Part model, mm, in its own coordinate system. Face numbers are marked on the shaded views. A direction names the side the tool comes from. Round coordinates to 2 decimals unless told otherwise and drop trailing zeros. Write each loop counter-clockwise with the first axis right and the second up, starting at its lowest first coordinate (ties: lowest second). Pieces come first, ordered by that corner, then holes.
1) Flat gauge pins, fed straight in: pin 1 (3 mm diameter, centred on x = 26.5, y = 5.5, fed in from +Z); pin 2 (2.5 mm diameter, centred on y = 7.5, z = 14.5, fed in from -X); pin 3 (2 mm diameter, centred on x = 33, y = 6, fed in from +Z). Where does each tip first touch, or does it go through?
2) Pull direction X, two halves, no side cores. Call the marked faces 1, 2 and 3: +X half, -X half, draft (parallel to the pull), parting line (faces both ways), or undercut.
3) Saw through at A-A on y = 6. Write the cut outline in (x, z), and give its area (3 significant figures).
4) Drill centre lines: L1, parallel to X at y = 6, z = 2.6; L2, parallel to X at y = 3.5, z = 14; L3, parallel to Y at x = 5, z = 3.2. Where is each one in solid material? Low to high.
5) Saw through at B-B on x = 31. Write the cut outline in (y, z).
6) Which spindle directions (+Z, -Z, +X, -X, +Y, -Y) get a long thin tool onto all of the face, cutting with end or side? Do the marked faces 4 and 5. Say none if no direction does.
7) Saw through at D-D on z = 2.75. Write the cut outline in (x, y).
8) Saw through at C-C on z = 14. Write the cut outline in (x, y).
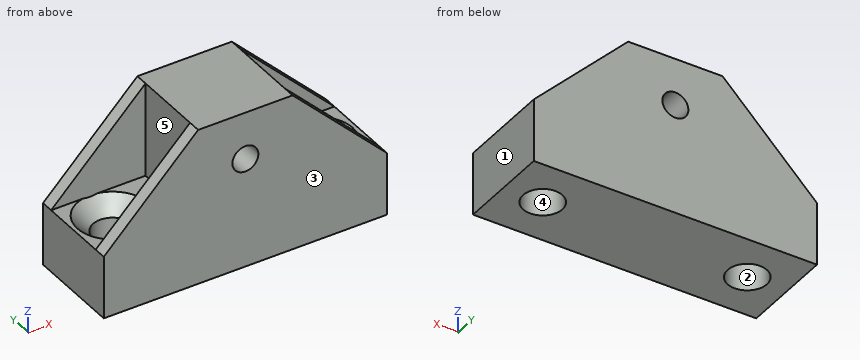
```python
from build123d import *

# Parameters (mm, degrees)
ESQUISSE1_W                  = 36
ESQUISSE1_H                  = 12
BOSS_EXTRU_1_DEPTH           = 8
ENL_V_MAT_EXTRU_1_DEPTH      = 39.781438859
ENL_V_MAT_EXTRU_1_DEPTH_BACK = 39.781438859
ESQUISSE2_R                  = 2.5
ESQUISSE3_W                  = 12
ESQUISSE3_H                  = 12
BOSS_EXTRU_2_DEPTH           = 12
ENL_V_MAT_EXTRU_2_DEPTH      = 43.895221179
ENL_V_MAT_EXTRU_2_DEPTH_BACK = 43.895221179
ESQUISSE4_R                  = 1.65
BOSS_EXTRU_3_DEPTH           = 1.6
BOSS_EXTRU_4_START           = -12
BOSS_EXTRU_4_DEPTH           = 1.6
CHANFREIN1_SIZE              = 2


with BuildPart() as part:
    # Esquisse1 → Boss.-Extru.1 (new body)
    with BuildSketch(Plane.XY):
        with Locations((18, 6)):
            Rectangle(ESQUISSE1_W, ESQUISSE1_H)
    extrude(amount=BOSS_EXTRU_1_DEPTH)

    # Esquisse2 → Enlèv. mat.-Extru.1 (cut, two sides: drawn at the far end of the back side and taken through both)
    with BuildSketch(Plane.XY.offset(8).offset(-ENL_V_MAT_EXTRU_1_DEPTH_BACK)):
        with Locations((5, 6)):
            Circle(ESQUISSE2_R)
        with Locations(Location((31, 6, 0), (0, 0, 180))):
            Circle(ESQUISSE2_R)
    extrude(amount=ENL_V_MAT_EXTRU_1_DEPTH + ENL_V_MAT_EXTRU_1_DEPTH_BACK, mode=Mode.SUBTRACT)

    # Esquisse3 → Boss.-Extru.2 (add)
    with BuildSketch(Plane(origin=(0, 12, 0), x_dir=(1, 0, 0), z_dir=(0, 1, 0))):
        with Locations((18, -14)):
            Rectangle(ESQUISSE3_W, ESQUISSE3_H)
    extrude(amount=-BOSS_EXTRU_2_DEPTH)

    # Esquisse4 → Enlèv. mat.-Extru.2 (cut, two sides: drawn at the far end of the back side and taken through both)
    with BuildSketch(Plane(origin=(0, 12, 0), x_dir=(1, 0, 0), z_dir=(0, 1, 0)).offset(-ENL_V_MAT_EXTRU_2_DEPTH_BACK)):
        with Locations(Location((18, -14, 0), (0, 0, 270))):
            Circle(ESQUISSE4_R)
    extrude(amount=ENL_V_MAT_EXTRU_2_DEPTH + ENL_V_MAT_EXTRU_2_DEPTH_BACK, mode=Mode.SUBTRACT)

    # Esquisse5 → Boss.-Extru.3 (add)
    with BuildSketch(Plane.XZ):
        Polygon((12, 8), (0, 8), (12, 20), align=None)
        Polygon((24, 20), (24, 8), (36, 8), align=None)
    extrude(amount=-BOSS_EXTRU_3_DEPTH)

    # Esquisse5<2> → Boss.-Extru.4 (add)
    with BuildSketch(Plane.XZ.offset(BOSS_EXTRU_4_START)):
        Polygon((12, 8), (0, 8), (12, 20), align=None)
        Polygon((24, 20), (24, 8), (36, 8), align=None)
    extrude(amount=BOSS_EXTRU_4_DEPTH)

    # Chanfrein1
    # the kernel refuses this chamfer: 2 mm, written as the material it takes off along each edge
    with BuildSketch(Plane(origin=(5, 6, 8), x_dir=(1, 0, 0), z_dir=(0, -1, 0))) as chanfrein1_piece_1_section:
        Polygon((2.5 + CHANFREIN1_SIZE, 0), (2.5, -CHANFREIN1_SIZE), (2.5, 0), align=None)
    chanfrein1_piece_1 = revolve(axis=Axis((5, 6, 8), (0, 0, 1)), mode=Mode.PRIVATE)
    chanfrein1_piece_1 = split(chanfrein1_piece_1, bisect_by=Plane(origin=(1.524895904, 1.6, 7.024895904), z_dir=(0, 1, 0)), keep=Keep.TOP, mode=Mode.PRIVATE)
    chanfrein1_piece_1 = split(chanfrein1_piece_1, bisect_by=Plane(origin=(1.524895904, 10.4, 7.024895904), z_dir=(0, -1, 0)), keep=Keep.TOP, mode=Mode.PRIVATE)
    add(chanfrein1_piece_1, mode=Mode.SUBTRACT)
    with BuildSketch(Plane(origin=(31, 6, 8), x_dir=(-1, 0, 0), z_dir=(0, 1, 0))) as chanfrein1_piece_2_section:
        Polygon((2.5 + CHANFREIN1_SIZE, 0), (2.5, -CHANFREIN1_SIZE), (2.5, 0), align=None)
    chanfrein1_piece_2 = revolve(axis=Axis((31, 6, 8), (0, 0, 1)), mode=Mode.PRIVATE)
    chanfrein1_piece_2 = split(chanfrein1_piece_2, bisect_by=Plane(origin=(34.475104096, 1.6, 7.024895904), z_dir=(0, 1, 0)), keep=Keep.TOP, mode=Mode.PRIVATE)
    chanfrein1_piece_2 = split(chanfrein1_piece_2, bisect_by=Plane(origin=(34.475104096, 10.4, 7.024895904), z_dir=(0, -1, 0)), keep=Keep.TOP, mode=Mode.PRIVATE)
    add(chanfrein1_piece_2, mode=Mode.SUBTRACT)


solid = part.part
```
Completed:
1. pin 1: stops at z = 8
1. pin 2: stops at x = 12
1. pin 3: stops at z = 6.5
2. face 1: +X half
2. face 2: undercut
2. face 3: draft
3. outline: (0, 0) - (2.5, 0) - (2.5, 6) - (0.5, 8) - (0, 8) - close; (7.5, 0) - (28.5, 0) - (28.5, 6) - (26.5, 8) - (24, 8) - (24, 20) - (12, 20) - (12, 8) - (9.5, 8) - (7.5, 6) - close; (33.5, 0) - (36, 0) - (36, 8) - (35.5, 8) - (33.5, 6) - close; hole circle Ø3.3 at (18, 14)
3. area: 335 mm2
4. L1: x = 0 to 2.5, 7.5 to 28.5, 33.5 to 36
4. L2: x = 12 to 16.35, 19.65 to 24
4. L3: y = 0 to 3.5, 8.5 to 12
5. outline: (0, 0) - (3.5, 0) - (3.5, 6) - (1.6, 7.9) - (1.6, 13) - (0, 13) - close; (8.5, 0) - (12, 0) - (12, 13) - (10.4, 13) - (10.4, 7.9) - (8.5, 6) - close
6. face 4: +Z, -Z
6. face 5: +Z, -X
7. outline: (0, 0) - (36, 0) - (36, 12) - (0, 12) - close; hole circle Ø5 at (5, 6); hole circle Ø5 at (31, 6)
8. outline: (6, 0) - (16.35, 0) - (16.35, 12) - (6, 12) - (6, 10.4) - (12, 10.4) - (12, 1.6) - (6, 1.6) - close; (19.65, 0) - (30, 0) - (30, 1.6) - (24, 1.6) - (24, 10.4) - (30, 10.4) - (30, 12) - (19.65, 12) - close
